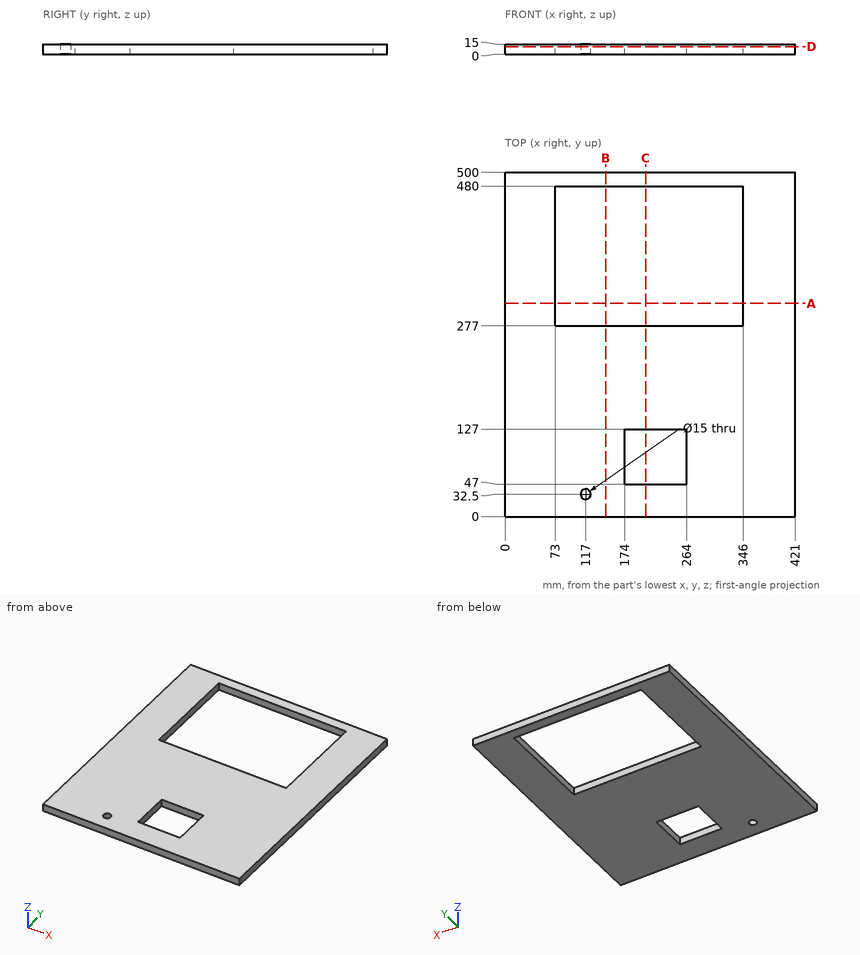
Verification items for this drawing (mm, ordinates from the low corner). Give positions to 0.01 mm unless a question says otherwise; leave off trailing zeros. Order: outer loops, then holes, each group sorted by start corner. A loop starts at its lowest first (then second) coordinate and runs counter-clockwise, first axis right, second up. Notation, with made-up numbers: M 52,49.25 L 61,49.25 A22 cw 61,56.25 Z; hole C 30,-0.75 d8. An arc over 180 degrees is marked long. Use a Markdown table: item, result.
Item 1: Section check C-C (x = 204). Record the cut outline in (y, z), and give its area (4 significant figures).
Answers follow:
| item | result |
|---|---|
| outline | M 0,0 L 47,0 L 47,15 L 0,15 Z; M 127,0 L 277,0 L 277,15 L 127,15 Z; M 480,0 L 500,0 L 500,15 L 480,15 Z |
| area | 3,255 mm2 |
Item 2: Section check B-B (x = 146). Record the cut outline in (y, z), and give its area (4 significant figures).
Answers follow:
| item | result |
|---|---|
| outline | M 0,0 L 277,0 L 277,15 L 0,15 Z; M 480,0 L 500,0 L 500,15 L 480,15 Z |
| area | 4,455 mm2 |
Item 3: Section check A-A (y = 309.5). Record the cut outline in (x, z).
Answers follow:
| item | result |
|---|---|
| outline | M 0,0 L 73,0 L 73,15 L 0,15 Z; M 346,0 L 421,0 L 421,15 L 346,15 Z |
Item 4: Section check D-D (z = 11). Record the cut outline in (x, y).
Answers follow:
| item | result |
|---|---|
| outline | M 0,0 L 421,0 L 421,500 L 0,500 Z; hole M 73,277 L 346,277 L 346,480 L 73,480 Z; hole C 117,32.5 d15; hole M 174,47 L 264,47 L 264,127 L 174,127 Z |
Item 5: Material ranges on line 1 along Y through (x, z) = (117, 6.75); line 2 along Y through (x, z) = (183.5, 1.25); line 3 along Y through (x, z) = (324, 9.5), recorded low to high.
Answers follow:
| item | result |
|---|---|
| line 1 | y = 0 to 25, 40 to 277, 480 to 500 |
| line 2 | y = 0 to 47, 127 to 277, 480 to 500 |
| line 3 | y = 0 to 277, 480 to 500 |
